Source: CAD feature listing. Evaluate the final solid. Frame: model axes, mm. Round coordinates to 2 decimals unless told otherwise and drop trailing zeros. Loops run counter-clockwise (first coordinate to the right, second up) from the corner with the lowest first, then second, coordinate; pieces in that order, holes last.
(1) Material intervals for probe 1 along X at (y, z) = (3, 1.3); probe 2 along X at (y, z) = (4.5, 1.1); probe 3 along Y at (x, z) = (24, 0.25), sorted ascending.
(2) First-contact query: pin 1 Ø3.5 at (x, y) = (24.36, 2.79) entering from -Z. Flat tip, straight axial feed; report the tip coordinate or a pass-through.
(3) Section B-B, the plane y = -17. Return the cut outline in (x, z), plus the area to 3 significant figures.
(4) Section A-A, the plane z = 1.5. Return the cut outline in (x, y) (3 decimals).
(5) Section C-C, the plane x = -46. Return the cut outline in (y, z).
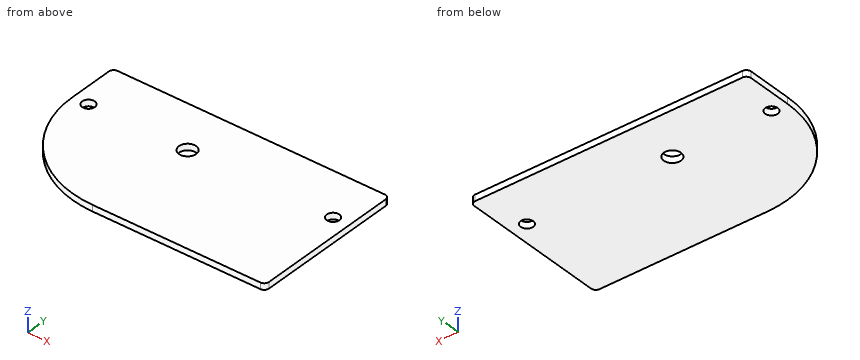
```python
from build123d import *

# Parameters (mm, degrees)
SKETCH1_W           = 117.069701218
SKETCH1_H           = 60.929458134
BOSS_EXTRUDE1_DEPTH = 2
SKETCH3_R           = 2
SKETCH3_R_2         = 2.75
CUT_EXTRUDE1_DEPTH  = 3


with BuildPart() as part:
    # Sketch1 → Boss-Extrude1 (new body)
    with BuildSketch(Plane.XY):
        Rectangle(SKETCH1_W, SKETCH1_H)
    extrude(amount=BOSS_EXTRUDE1_DEPTH)

    # Sketch3 → Cut-Extrude1 (cut, through all)
    with BuildSketch(Plane(origin=(0, 0, 0), x_dir=(-1, 0, 0), z_dir=(0, 0, -1))):
        with Locations((-24.357544508, 2.794584929)):
            Circle(SKETCH3_R)
        with Locations((53.534850609, 2.794584929)):
            Circle(SKETCH3_R)
        with Locations((21.97485305, 2.79526544)):
            Circle(SKETCH3_R_2)
        with BuildLine():
            Line((25.349937795, -30.464729067), (25.349937795, -36.756710317))
            Line((25.349937795, -36.756710317), (60.494221028, -36.756710317))
            Line((60.494221028, -36.756710317), (60.494221028, 2.79526544))
            Line((60.494221028, 2.79526544), (58.534850609, 2.79526544))
            ThreePointArc((58.534850609, 2.79526544), (48.841775064, -20.718537892), (25.349937795, -30.464729067))
        make_face()
        with BuildLine():
            Line((-29.591361368, 17.035270933), (-29.591361368, -28.964729067))
            ThreePointArc((-29.591361368, -28.964729067), (-29.15202154, -30.025389239), (-28.091361368, -30.464729067))
            Line((-28.091361368, -30.464729067), (-58.534850609, -30.464729067))
            Line((-58.534850609, -30.464729067), (-58.534850609, 30.464729067))
            Line((-58.534850609, 30.464729067), (58.534850609, 30.464729067))
            Line((58.534850609, 30.464729067), (58.534850609, 17.035270933))
            ThreePointArc((58.534850609, 17.035270933), (58.095510781, 18.095931105), (57.034850609, 18.535270933))
            Line((57.034850609, 18.535270933), (-28.091361368, 18.535270933))
            ThreePointArc((-28.091361368, 18.535270933), (-29.15202154, 18.095931105), (-29.591361368, 17.035270933))
        make_face()
    extrude(amount=-CUT_EXTRUDE1_DEPTH, mode=Mode.SUBTRACT)


solid = part.part
```
Output values:
1. probe 1: x = -58.53 to -55.52, -51.55 to -24.72, -19.23 to 22.37, 26.35 to 29.59
1. probe 2: x = -58.53 to -54.58, -52.49 to -24.13, -19.82 to 23.31, 25.4 to 29.59
1. probe 3: y = -30.46 to 0.83, 4.76 to 18.54
2. pin 1: passes through
3. outline: (-52.04, 0) - (29.59, 0) - (29.59, 2) - (-52.04, 2) - close
3. area: 163 mm2
4. outline: (-58.535, 2.645) arc R33.185 ccw to (-25.35, -30.465) - (28.091, -30.465) arc R1.5 ccw to (29.591, -28.965) - (29.591, 17.035) arc R1.5 ccw to (28.091, 18.535) - (-57.035, 18.535) arc R1.5 ccw to (-58.535, 17.035) - close; hole circle Ø4 at (-53.535, 2.795); hole circle Ø5.5 at (-21.975, 2.795); hole circle Ø4 at (24.358, 2.795)
5. outline: (-23.26, 0) - (18.54, 0) - (18.54, 2) - (-23.26, 2) - close
